```python
from build123d import *

# Parameters (mm, degrees)
F2_R          = 2
F3_DEPTH      = 12.701
F3_DEPTH_BACK = 12.701
F4_R          = 2
F5_DEPTH      = 10.0010001
F6_R          = 1.5875
F7_DEPTH      = 10.001


with BuildPart() as f1:
    # F0 (on Front) → F1 (revolve)
    with BuildSketch(Plane.XZ):
        Polygon((0, 6), (0, 0), (10, 0), (10, 12.7), (6, 12.7), (6, 6), align=None)
    revolve(axis=Axis((5, 0, 0), (-1, 0, 0)))

    # F2 (on Top) → F3 (cut, two sides)
    with BuildSketch(Plane.XY) as f3_sk:
        with Locations((3, 0)):
            Circle(F2_R)
    extrude(amount=-F3_DEPTH, mode=Mode.SUBTRACT)
    extrude(f3_sk.sketch, amount=F3_DEPTH_BACK, mode=Mode.SUBTRACT)

    # F4 (on face) → F5 (cut, through all)
    with BuildSketch(Plane.YZ.offset(10)):
        with Locations((0, 9)):
            Circle(F4_R)
        with Locations((9, 0)):
            Circle(F4_R)
        with Locations((0, -9)):
            Circle(F4_R)
        with Locations((-9, 0)):
            Circle(F4_R)
    extrude(amount=-F5_DEPTH, mode=Mode.SUBTRACT)

    # F6 (on face) → F7 (cut, through all)
    with BuildSketch(Plane(origin=(0, 0, 0), x_dir=(0, -1, 0), z_dir=(-1, 0, 0))):
        Circle(F6_R)
    extrude(amount=-F7_DEPTH, mode=Mode.SUBTRACT)


solid = f1.part
```
Geometry check sheet. Reference: the model listing, model coordinates, mm. Round coordinates to 2 decimals unless told otherwise and drop trailing zeros. Order: outer loops, then holes, each group sorted by start corner. A loop starts at its lowest first (then second) coordinate and runs counter-clockwise, first axis right, second up. Notation, with made-up numbers: (46.25, 57.25) - (96.25, 57.25) arc R11 ccw to (96.25, 68.25) - close; hole circle Ø2 at (-40, -28.75). An arc over 180 degrees is marked (long way). Use a Markdown table: item, result. Add a question column.
(1) Sectioned sample at D-D, the plane x = 3. Enter the section's corners in (y, z).
(2) Depth check by flat-ended pin: pin 1 (1.5 mm diameter, centred on x = 5.5, z = -4.5, fed in from +Y); pin 2 (5 mm diameter, centred on x = 3, y = 0, fed in from -Z); pin 3 (2 mm diameter, centred on x = 7.5, y = 3, fed in from +Z); pin 4 (2.5 mm diameter, centred on y = 9, z = 0, fed in from -X). Enter the tip coordinate at first touch or a pass-through.
(3) Release check for a two-part mould opening along Z. For faces 1 (the cylindrical face through (2.96, -2.3, 5.54)), 2 (the flat face through (6, 3, 5.5)), 3 (the cylindrical face through (0.681, -1.514, 0.477)), 4 (the cylindrical face through (8, 7, 0)) record: pulls with the +Z half, pulls with the -Z half, needs draft (parallel to the pull), parting line crosses it, or undercut.
(4) Material ranges on line 1 along X through (y, z) = (0, 4); line 2 along Z through (x, y) = (0.65, 0); line 3 along X through (y, z) = (7.5, 5.25), recorded low to high. Write a range as [from, to].
(5) Sectioned sample at C-C, the plane y = -9. Enter the section's corners in (x, z), and give its area (3 significant figures).
(6) Sectioned sample at B-B, the plane z = 4.75. Enter the section's corners in (x, y), and give its area (3 significant figures).
(7) Sectioned sample at A-A, the plane y = 0. Enter the section's corners in (x, z), and give its area (4 significant figures).
Answers below:
| question | item | result |
|---|---|---|
| 1 | outline | (-2, -5.66) - (-2, 5.66) arc R6 ccw to start; (2, -5.66) arc R6 ccw to (2, 5.66) - close |
| 2 | pin 1 | y = 12.07 |
| 2 | pin 2 | z = -6 |
| 2 | pin 3 | z = 12.54 |
| 2 | pin 4 | through |
| 3 | face 1 | parting line crosses it |
| 3 | face 2 | needs draft |
| 3 | face 3 | undercut |
| 3 | face 4 | undercut |
| 4 | line 1 | [0, 1], [5, 10] |
| 4 | line 2 | [-6, -1.59], [1.59, 6] |
| 4 | line 3 | [6, 10] |
| 5 | outline | (6, -8.96) - (10, -8.96) - (10, -2) - (6, -2) - close; (6, 2) - (10, 2) - (10, 8.96) - (6, 8.96) - close |
| 5 | area | 55.7 mm² |
| 6 | outline | (0, -3.67) - (6, -3.67) - (6, -11.78) - (10, -11.78) - (10, 11.78) - (6, 11.78) - (6, 3.67) - (0, 3.67) - close; hole circle Ø4 at (3, 0) |
| 6 | area | 126 mm² |
| 7 | outline | (0, -6) - (1, -6) - (1, -1.59) - (0, -1.59) - close; (0, 1.59) - (1, 1.59) - (1, 6) - (0, 6) - close; (5, -6) - (6, -6) - (6, -7) - (10, -7) - (10, -1.59) - (5, -1.59) - close; (5, 1.59) - (10, 1.59) - (10, 7) - (6, 7) - (6, 6) - (5, 6) - close; (6, -12.7) - (10, -12.7) - (10, -11) - (6, -11) - close; (6, 11) - (10, 11) - (10, 12.7) - (6, 12.7) - close |
| 7 | area | 74.55 mm² |
